```python
from build123d import *

# Parameters (mm, degrees)
F1_R          = 2.5
F1_R_2        = 2.15
F2_DEPTH      = 50
F2_DEPTH_BACK = 50
F0_W          = 45
F0_H          = 2
F6_DEPTH      = 50.001
F6_DEPTH_BACK = 50.0631497295
F7_DEPTH      = 100.001


with BuildPart() as f2:
    # F1 (on Top) → F2 (new body, two sides)
    with BuildSketch(Plane.XY) as f2_sk:
        Circle(F1_R)
        Circle(F1_R_2, mode=Mode.SUBTRACT)
    extrude(amount=F2_DEPTH)
    extrude(f2_sk.sketch, amount=-F2_DEPTH_BACK)

    # F0 (on Front) → F3 (revolve)
    with BuildSketch(Plane.XZ):
        with Locations((22.5, -16)):
            Rectangle(F0_W, F0_H)
        with Locations((22.5, 44)):
            Rectangle(F0_W, F0_H)
        with Locations((22.5, -12)):
            Rectangle(F0_W, F0_H)
        with Locations((22.5, -32)):
            Rectangle(F0_W, F0_H)
        with Locations((22.5, -36)):
            Rectangle(F0_W, F0_H)
        with Locations((22.5, -44)):
            Rectangle(F0_W, F0_H)
        with Locations((22.5, 12)):
            Rectangle(F0_W, F0_H)
        with Locations((22.5, 32)):
            Rectangle(F0_W, F0_H)
        with Locations((22.5, 40)):
            Rectangle(F0_W, F0_H)
        with Locations((22.5, 24)):
            Rectangle(F0_W, F0_H)
        with Locations((22.5, 28)):
            Rectangle(F0_W, F0_H)
        with Locations((22.5, 4)):
            Rectangle(F0_W, F0_H)
        with Locations((22.5, 16)):
            Rectangle(F0_W, F0_H)
        with Locations((22.5, 8)):
            Rectangle(F0_W, F0_H)
        with Locations((22.5, -28)):
            Rectangle(F0_W, F0_H)
        with Locations((22.5, -24)):
            Rectangle(F0_W, F0_H)
        with Locations((22.5, -20)):
            Rectangle(F0_W, F0_H)
        with Locations((22.5, -8)):
            Rectangle(F0_W, F0_H)
        with Locations((22.5, -4)):
            Rectangle(F0_W, F0_H)
        with Locations((22.5, 20)):
            Rectangle(F0_W, F0_H)
        with Locations((22.5, 36)):
            Rectangle(F0_W, F0_H)
        with Locations((22.5, -40)):
            Rectangle(F0_W, F0_H)
        with Locations((22.5, -48)):
            Rectangle(F0_W, F0_H)
        with Locations((22.5, 48)):
            Rectangle(F0_W, F0_H)
        with Locations((22.5, 0)):
            Rectangle(F0_W, F0_H)
    revolve(axis=Axis((0, 0, 0), (0, 0, -1)))

    # F4 (on Front) → F5 (revolve)
    with BuildSketch(Plane.XZ):
        Polygon((5, 50.0621497295), (0, 50.0621497295), (0, -49.9378502705), (15, -49.9378502705), align=None)
    revolve(axis=Axis((0, 0, 0.0621497295), (0, 0, -1)))

    # F1 (on Top) → F6 (cut, two sides)
    with BuildSketch(Plane.XY) as f6_sk:
        Circle(F1_R)
        Circle(F1_R_2, mode=Mode.SUBTRACT)
    extrude(amount=-F6_DEPTH, mode=Mode.SUBTRACT)
    extrude(f6_sk.sketch, amount=F6_DEPTH_BACK, mode=Mode.SUBTRACT)

    # F7 (cut, through all): a face of the model
    f7_faces = [f2.faces().sort_by_distance(p)[0] for p in [
        (0, 0, 50.0621497295),
    ]]
    extrude(f7_faces, amount=-F7_DEPTH, mode=Mode.SUBTRACT)


solid = f2.part
```
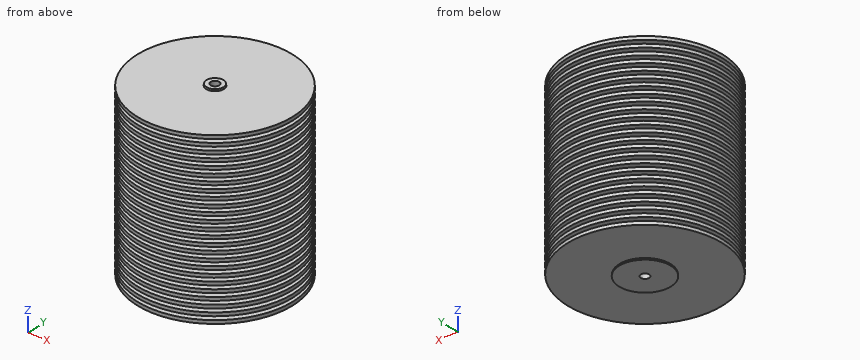
The listing builds one solid part. Answer for the finished solid, in the listing's coordinates (mm). Give positions to 0.01 mm unless a question says otherwise; leave off trailing zeros. One line per item, written item: value.
Q1. Find the intervals of material crossed by line 1 (X direction, y = 0, z = 36); line 2 (X direction, y = -7, z = -5.5), in increasing order. Write a range as from..to.
Working result:
line 1: x = -45..-2.5, 2.5..45
line 2: x = -7.9..7.9
Q2. Flat-ended cylindrical pins translate along their axes: P1, Ø1.5, axis at x = 25.5, y = -5.5, coming from the -Z side; P2, Ø2, axis at x = -26, z = 13.5, coming from the -Y side; P3, Ø2, axis at x = -3, z = 30.5, coming from the -Y side. Find the tip coordinate at first contact, or state that the pin passes through.
Working result:
P1: stops at z = -49
P2: stops at y = -37.33
P3: stops at y = -44.95
Q3. A cutting plane is placed at A-A on x = -31. Give the number of separate pieces and of enclosed holes in the cut face, then the cut area to 3 significant figures.
Working result:
separate pieces: 25
enclosed holes: 0
area: 3,260 mm^2
